Can you work these out from the model? Positions are in its coordinate system, mm. Face numbers are marked on the shaded views. A direction names the side the tool comes from. Give positions to 0.01 mm unless a question says otherwise; leave off trailing zeros. Order: outer loops, then holes, each group sorted by start corner. A loop starts at its lowest first (then second) coordinate and runs counter-clockwise, first axis right, second up. Notation, with made-up numbers: M 48.25,-5.75 L 58.25,-5.75 A24 ccw 58.25,32.25 Z; hole C 37,64.5 d7. An arc over 180 degrees is marked long. Write each question's results on one line, items separated by ' | '.
from build123d import *

# Parameters (mm, degrees)
F0_R     = 101.6
F2_DEPTH = 25.4
F1_R     = 12.7
F3_DEPTH = 25.401
F5_DEPTH = 25.401
F6_SIZE  = 3.175


with BuildPart() as f2:
    # F0 (on Front) → F2 (new body)
    with BuildSketch(Plane.XZ):
        Circle(F0_R)
    extrude(amount=F2_DEPTH)

    # F1 (on Front) → F3 (cut, through all)
    with BuildSketch(Plane.XZ):
        Circle(F1_R)
    extrude(amount=F3_DEPTH, mode=Mode.SUBTRACT)

    # F4 (on face) → F5 (cut, through all)
    with BuildSketch(Plane.XZ.offset(25.4)):
        with BuildLine():
            ThreePointArc((22.225, 38.494829), (38.494829, 22.225), (44.45, 0))
            ThreePointArc((44.45, 0), (57.15, -12.7), (69.85, 0))
            ThreePointArc((69.85, 0), (60.491874, 34.925), (34.925, 60.491874))
            ThreePointArc((34.925, 60.491874), (17.576477, 55.843352), (22.225, 38.494829))
        make_face()
        with BuildLine():
            ThreePointArc((-44.45, 0), (-38.494829, 22.225), (-22.225, 38.494829))
            ThreePointArc((-22.225, 38.494829), (-17.576477, 55.843352), (-34.925, 60.491874))
            ThreePointArc((-34.925, 60.491874), (-60.491874, 34.925), (-69.85, 0))
            ThreePointArc((-69.85, 0), (-57.15, -12.7), (-44.45, 0))
        make_face()
        with BuildLine():
            ThreePointArc((22.225, -38.494829), (0, -44.45), (-22.225, -38.494829))
            ThreePointArc((-22.225, -38.494829), (-39.573523, -43.143352), (-34.925, -60.491874))
            ThreePointArc((-34.925, -60.491874), (0, -69.85), (34.925, -60.491874))
            ThreePointArc((34.925, -60.491874), (39.573523, -43.143352), (22.225, -38.494829))
        make_face()
    extrude(amount=-F5_DEPTH, mode=Mode.SUBTRACT)

    # F6
    f6_edges = [f2.edges().sort_by_distance(p)[0] for p in [
        (-101.6, -25.4, 0),
        (-60.491874, -25.4, 34.925),
        (38.494829, -25.4, 22.225),
        (0, -25.4, -44.45),
    ]]
    chamfer(f6_edges, length=F6_SIZE)


solid = f2.part
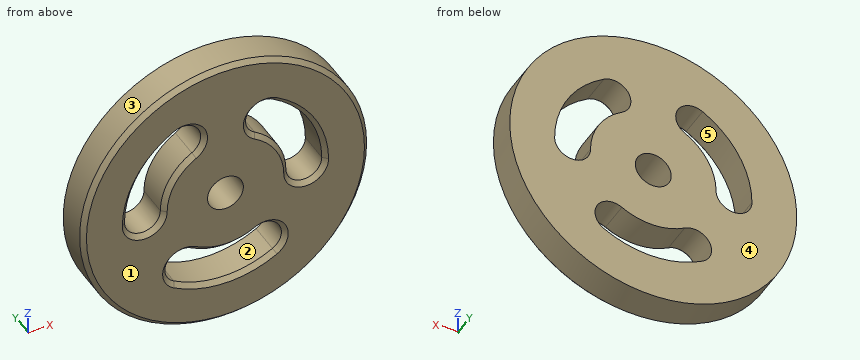
(1) We'd pull the mould along Z, two halves only. Please class the marked faces 3, 4 and 5: +Z half, -Z half, draft (parallel to the pull), parting line (faces both ways), or undercut.
Data:
face 3: parting line | face 4: draft | face 5: undercut
(2) Will these pins go through, and if not, where does the flat tip stop? P1, Ø1.5, axis at y = -17.5, z = -27.5, coming from the +X side; P2, Ø2, axis at y = -5, z = -65, coming from the +X side; P3, Ø10, axis at y = -11, z = -76.5, coming from the +X side.
Data:
P1: stops at x = 98.02 | P2: stops at x = 78.91 | P3: stops at x = 72.18
(3) For the marked faces 1 and 2, which set-ups out of +Z, -Z, +X, -X, +Y, -Y let a thin tool reach every point of the face, with its end or its side?
Data:
face 1: +Z, -Z, +X, -X, -Y | face 2: +Y, -Y
(4) Imagine slicing it at B-B, the plane y = -10.25. Write out the boundary of the cut face in (x, z) (3 decimals).
Data:
outline: C 0,0 d203.2; hole M -69.85,0 A12.7 ccw -44.45,0 A44.45 cw -22.225,38.495 A12.7 ccw -34.925,60.492 A69.85 ccw Z; hole M -34.925,-60.492 A69.85 ccw 34.925,-60.492 A12.7 ccw 22.225,-38.495 A44.45 cw -22.225,-38.495 A12.7 ccw Z; hole C 0,0 d25.4; hole M 22.225,38.495 A44.45 cw 44.45,0 A12.7 ccw 69.85,0 A69.85 ccw 34.925,60.492 A12.7 ccw Z
(5) Imagine slicing it at C-C, the plane z = 29. Count the separate pieces of the cut face and the enclosed holes in it, plus the area to 3 significant figures.
Data:
separate pieces: 3 | enclosed holes: 0 | area: 3,390 mm2
(6) Imagine slicing it at A-A, the plane x = 0. Write out the boundary of the cut face in (y, z) (3 decimals).
Data:
outline: M -25.4,-98.425 L -22.225,-101.6 L 0,-101.6 L 0,-69.85 L -22.225,-69.85 L -25.4,-73.025 Z; M -25.4,-41.275 L -22.225,-44.45 L 0,-44.45 L 0,-12.7 L -25.4,-12.7 Z; M -25.4,12.7 L 0,12.7 L 0,101.6 L -22.225,101.6 L -25.4,98.425 Z
(7) I need wall thicknesses on L1, parallel to Z at x = 0, y = -19.25; L2, parallel to X at y = -13.5, z = 50; L3, parallel to Z at x = 33, y = -20.25. Which ranges of each line are inside material? Lowest first, please. Write a range as from..to.
Data:
L1: z = -101.6..-69.85, -44.45..-12.7, 12.7..101.6 | L2: x = -88.45..-48.78, -15.89..15.89, 48.78..88.45 | L3: z = -96.09..-61.56, -37.59..29.78, 61.4..96.09
